```python
from build123d import *

# Parameters (mm, degrees)
SKETCH1_W           = 40
SKETCH1_H           = 35
BOSS_EXTRUDE1_DEPTH = 6
SKETCH2_R           = 2.5
CUT_EXTRUDE1_DEPTH  = 6
SKETCH3_W           = 20
SKETCH3_H           = 35
BOSS_EXTRUDE2_DEPTH = 4
SKETCH4_W           = 18
SKETCH4_H           = 35
CUT_EXTRUDE2_DEPTH  = 6
FILLET2_R           = 4
FILLET3_R           = 4


with BuildPart() as part:
    # Sketch1 → Boss-Extrude1 (new body)
    with BuildSketch(Plane(origin=(0, 0, 0), x_dir=(1, 0, 0), z_dir=(0, 1, 0))):
        with Locations((7.786458333, -9.114583333)):
            Rectangle(SKETCH1_W, SKETCH1_H)
    extrude(amount=BOSS_EXTRUDE1_DEPTH)

    # Sketch2 → Cut-Extrude1 (cut)
    with BuildSketch(Plane(origin=(0, 6, 0), x_dir=(1, 0, 0), z_dir=(0, 1, 0))):
        with Locations(Location((-7.213541667, -21.614583333, 0), (0, 0, 270))):
            Circle(SKETCH2_R)
        with Locations(Location((22.786458333, 3.385416667, 0), (0, 0, 270))):
            Circle(SKETCH2_R)
        with Locations(Location((22.786458333, -21.614583333, 0), (0, 0, 270))):
            Circle(SKETCH2_R)
        with Locations(Location((-7.213541667, 3.385416667, 0), (0, 0, 270))):
            Circle(SKETCH2_R)
    extrude(amount=-CUT_EXTRUDE1_DEPTH, mode=Mode.SUBTRACT)

    # Sketch3 → Boss-Extrude2 (add)
    with BuildSketch(Plane(origin=(0, 6, 0), x_dir=(1, 0, 0), z_dir=(0, 1, 0))):
        with Locations((7.786458333, -9.114583333)):
            Rectangle(SKETCH3_W, SKETCH3_H)
    extrude(amount=BOSS_EXTRUDE2_DEPTH)

    # Sketch4 → Cut-Extrude2 (cut)
    with BuildSketch(Plane.XZ):
        with Locations((7.786458333, 9.114583333)):
            Rectangle(SKETCH4_W, SKETCH4_H)
    extrude(amount=-CUT_EXTRUDE2_DEPTH, mode=Mode.SUBTRACT)

    # Fillet2
    fillet2_edges = [part.edges().sort_by_distance(p)[0] for p in [
        (-1.213541667, 6, 9.114583333),
        (16.786458333, 6, 9.114583333),
    ]]
    fillet(fillet2_edges, radius=FILLET2_R)

    # Fillet3
    fillet3_edges = [part.edges().sort_by_distance(p)[0] for p in [
        (17.786458333, 10, 9.114583333),
        (-2.213541667, 10, 9.114583333),
    ]]
    fillet(fillet3_edges, radius=FILLET3_R - 0.0001)  # a hair under: the kernel refuses the full size


solid = part.part
```
Input: part model. Units: mm. Frame: model coordinates. A direction names the side the tool comes from. Coordinates: 2 decimals unless noted, no trailing zeros. Loops run counter-clockwise (first coordinate to the right, second up) from the corner with the lowest first, then second, coordinate; pieces in that order, holes last.
Q1. Section D-D, the plane y = 0.5. Return the cut outline in (x, z).
Results are:
outline: (-12.21, -8.39) - (-1.21, -8.39) - (-1.21, 26.61) - (-12.21, 26.61) - close; (16.79, -8.39) - (27.79, -8.39) - (27.79, 26.61) - (16.79, 26.61) - close; hole circle Ø5 at (-7.21, -3.39); hole circle Ø5 at (-7.21, 21.61); hole circle Ø5 at (22.79, -3.39); hole circle Ø5 at (22.79, 21.61)
Q2. Mould query, pull axis X, two halves, no side actions, for faces 1 (the cylindrical face through (-8.735, 3.042, 19.631)), 2 (the flat face through (22, 0, 9)), 3 (the flat face through (8, 6, 9)), 4 (the flat face through (27.786, 3, 9)). Classes: +X half, -X half, draft (parallel to the pull), parting line (faces both ways), or undercut.
Results are:
face 1: undercut
face 2: draft
face 3: undercut
face 4: +X half
Q3. Set-up query: faces 5 (the flat face through (8, 7, 26.615)), 6 (the cylindrical face through (-0.07, 4.8, 9.36)), 7 (the flat face through (-7, 6, 9)). Return all of +Z, -Z, +X, -X, +Y, -Y with unobstructed straight access to the full face (end or side cutting, diameter ignored); none if empty.
Results are:
face 5: +Z, +X, -X, +Y, -Y
face 6: +Z, -Z, -Y
face 7: +Z, -Z, -X, +Y
Q4. Section B-B, the plane z = 22.5. Give the number of separate pieces and of enclosed holes in the cut face, and give its area (3 significant figures).
Results are:
separate pieces: 3
enclosed holes: 0
area: 156 mm2
Q5. Section A-A, the plane y = 4.75. Return the cut outline in (x, z).
Results are:
outline: (-12.21, -8.39) - (-0.12, -8.39) - (-0.12, 26.61) - (-12.21, 26.61) - close; (15.69, -8.39) - (27.79, -8.39) - (27.79, 26.61) - (15.69, 26.61) - close; hole circle Ø5 at (-7.21, -3.39); hole circle Ø5 at (-7.21, 21.61); hole circle Ø5 at (22.79, -3.39); hole circle Ø5 at (22.79, 21.61)
Q6. Contact query for flat-ended pins moving along their axis: pin 1 (8 mm diameter, centred on x = -8, z = 14, fed in from +Y); pin 2 (2 mm diameter, centred on x = 0, z = 22.5, fed in from +Y); pin 3 (1 mm diameter, centred on x = 15, z = 7.5, fed in from -Y). Output: stop coordinate, or through.
Results are:
pin 1: stops at y = 6
pin 2: stops at y = 9.92
pin 3: stops at y = 4.94
Q7. Line query: line 1 along X through (y, z) = (1.5, 1); line 2 along Y through (x, z) = (4, 6.5); line 3 along Z through (x, y) = (-6, 2.25). Output: solid intervals per line, ascending.
Results are:
line 1: x = -12.21 to -1.21, 16.79 to 27.79
line 2: y = 6 to 10
line 3: z = -8.39 to -5.57, -1.2 to 19.43, 23.8 to 26.61
Q8. Section C-C, the plane x = -9. Return the cut outline in (y, z).
Results are:
outline: (0, -8.39) - (6, -8.39) - (6, -5.13) - (0, -5.13) - close; (0, -1.64) - (6, -1.64) - (6, 19.87) - (0, 19.87) - close; (0, 23.36) - (6, 23.36) - (6, 26.61) - (0, 26.61) - close
